```python
from build123d import *

# Parameters (mm, degrees)
F0_W     = 150
F0_H     = 150
F0_R     = 3
F1_DEPTH = 7
F2_R     = 5
F3_DEPTH = 17.5


with BuildPart() as f1:
    # F0 (on Front) → F1 (new body)
    with BuildSketch(Plane.XZ):
        with Locations((6.393103, 60.418246)):
            Rectangle(F0_W, F0_H)
        with Locations((-60.606897, -6.581754)):
            Circle(F0_R, mode=Mode.SUBTRACT)
        with Locations((73.393103, -6.581754)):
            Circle(F0_R, mode=Mode.SUBTRACT)
        with Locations((-60.606897, 60.418246)):
            Circle(F0_R, mode=Mode.SUBTRACT)
        with Locations((6.393103, 127.418246)):
            Circle(F0_R, mode=Mode.SUBTRACT)
    extrude(amount=F1_DEPTH)

    # F2 (on face) → F3 (join)
    with BuildSketch(Plane.XZ.offset(7)):
        with Locations((-56.816334, 123.454368)):
            Circle(F2_R)
        with Locations((-13.816334, 123.454368)):
            Circle(F2_R)
        with Locations((-58.237764, 76.475867)):
            Circle(F2_R)
        with Locations((-43.606897, 0.418246)):
            Circle(F2_R)
        with Locations((20.157204, 68.235859)):
            Circle(F2_R)
        with Locations((60.537563, 97.721901)):
            Circle(F2_R)
    extrude(amount=F3_DEPTH)


solid = f1.part
```
CAD build for the part. Positions are in the model's coordinates, mm. A direction names the side the tool comes from. Round coordinates to 2 decimals unless told otherwise and drop trailing zeros. Loops run counter-clockwise (first coordinate to the right, second up) from the corner with the lowest first, then second, coordinate; pieces in that order, holes last. Notation, with made-up numbers: (60, 20.25) - (103, 20.25) arc R18 cw to (103, 24.25) - close; hole circle Ø5 at (-3.75, -30.75). An arc over 180 degrees is marked (long way). Return JSON: item names as keys, results as strings. Group by question number.
Q1. Band-saw the part on D-D on x = 12. Give the cut face in (y, z), plus the area to 3 significant figures.
Q2. Band-saw the part on A-A on x = -43. Give the cut face in (y, z), plus the area to 3 significant figures.
Q3. Drill centre lines: line 1 along Y through (x, z) = (-54, 13.5); line 2 along Z through (x, y) = (-43.5, -22.5); line 3 along X through (y, z) = (-19.25, 0.5). Where is each one in solid material? Low to high. Write a range as [from, to].
Q4. Band-saw the part on C-C on z = 104.5. Give the cut face in (x, y).
Q5. Two-plate mould, pull along Z, no slides. Class faces 3 (the face through (-11.13, -15.63, 127.67)), 4 (the face through (-57.47, -15.63, 128.41)), 5 (the face through (60, -24.5, 98)): +Z half, -Z half, draft (parallel to the pull), parting line (faces both ways), or undercut.
Q6. Band-saw the part on B-B on y = -14.75. Give the cut face in (x, z), plus the area to 3 significant figures.
Q7. Tool access for faces 1 (the face through (5, -7, 61)), 2 (the face through (5, -3, -14.582)): list every direction of +Z, -Z, +X, -X, +Y, -Y with a clear straight run to the whole face (end or side of a thin tool).
Q8. Flat gauge pins, fed straight in: pin 1 Ø3 at (x, y) = (17, -16.5) entering from +Z; pin 2 Ø2 at (y, z) = (-11.5, 115.5) entering from -X; pin 3 Ø8 at (x, y) = (55, -12.5) entering from +Z; pin 4 Ø3 at (x, z) = (33, 30.5) entering from -Y. Where does each tip first touch, or does it go through?
Solutions:
{
 "1": {"outline": "(-7, -14.58) - (0, -14.58) - (0, 135.42) - (-7, 135.42) - close", "area": "1,050 mm^2"},
 "2": {"outline": "(-24.5, -4.54) - (-7, -4.54) - (-7, -14.58) - (0, -14.58) - (0, 135.42) - (-7, 135.42) - (-7, 5.38) - (-24.5, 5.38) - close", "area": "1,220 mm^2"},
 "3": {"line 1": "y = [-7, 0]", "line 2": "z = [-4.58, 5.42]", "line 3": "x = [-48.61, -38.61]"},
 "4": {"outline": "(-68.61, -7) - (81.39, -7) - (81.39, 0) - (-68.61, 0) - close"},
 "5": {"face 3": "parting line", "face 4": "undercut", "face 5": "draft"},
 "6": {"outline": "circle Ø10 at (-58.24, 76.48); circle Ø10 at (-56.82, 123.45); circle Ø10 at (-43.61, 0.42); circle Ø10 at (-13.82, 123.45); circle Ø10 at (20.16, 68.24); circle Ø10 at (60.54, 97.72)", "area": "471 mm^2"},
 "7": {"face 1": "-Y", "face 2": "-Z, +X, -X, +Y, -Y"},
 "8": {"pin 1": "stops at z = 72.95", "pin 2": "passes through", "pin 3": "stops at z = 102.48", "pin 4": "stops at y = -7"}
}
